```python
from build123d import *


with BuildPart() as part:
    # Sketch 1 → Revolve 1 (revolve)
    with BuildSketch(Plane.XY, mode=Mode.PRIVATE) as revolve_1_sk:
        with BuildLine():
            Line((18.75, 20), (18.75, 24))
            ThreePointArc((18.75, 24), (18.457106781, 24.707106781), (17.75, 25))
            Line((17.75, 25), (-16, 25))
            ThreePointArc((-16, 25), (-16.258819045, 24.965925826), (-16.5, 24.866025404))
            Line((-16.5, 24.866025404), (-18.25, 23.855662433))
            ThreePointArc((-18.25, 23.855662433), (-18.616025404, 23.489637029), (-18.75, 22.989637029))
            Line((-18.75, 22.989637029), (-18.75, 19.1))
            ThreePointArc((-18.75, 19.1), (-18.457106781, 18.392893219), (-17.75, 18.1))
            Line((-17.75, 18.1), (-16, 18.1))
            Line((-16, 18.1), (-16, 20))
            Line((-16, 20), (18.75, 20))
        make_face()
    revolve(revolve_1_sk.sketch.rotate(Axis((-18.75, 0, 0), (1, 0, 0)), 90), axis=Axis((-18.75, 0, 0), (1, 0, 0)))


solid = part.part
```
Could you check a few things on this model? Use its own coordinates, in mm. A direction names the side the tool comes from. Give positions to 0.01 mm unless a question says otherwise; leave off trailing zeros. Write each loop counter-clockwise with the first axis right and the second up, starting at its lowest first coordinate (ties: lowest second). Pieces come first, ordered by that corner, then holes. Notation, with made-up numbers: (50, 44) -> (78, 44) arc R12 ccw to (78, 66) -> close; hole circle Ø1 at (52, 68.25). An arc over 180 degrees is marked (long way). Write each question's results on one line, items separated by ' | '.
1. I want a section at A-A, the plane z = 0. Write out the boundary of the cut face in (x, y), then the cut area to 3 significant figures.
Check sheet entries:
outline: (-18.75, -22.99) arc R1 ccw to (-18.25, -23.86) -> (-16.5, -24.87) arc R1 ccw to (-16, -25) -> (17.75, -25) arc R1 ccw to (18.75, -24) -> (18.75, -20) -> (-16, -20) -> (-16, -18.1) -> (-17.75, -18.1) arc R1 ccw to (-18.75, -19.1) -> close; (-18.75, 19.1) arc R1 ccw to (-17.75, 18.1) -> (-16, 18.1) -> (-16, 20) -> (18.75, 20) -> (18.75, 24) arc R1 ccw to (17.75, 25) -> (-16, 25) arc R1 ccw to (-16.5, 24.87) -> (-18.25, 23.86) arc R1 ccw to (-18.75, 22.99) -> close | area: 381 mm²
2. Will these pins go through, and if not, where does the flat tip stop? pin 1 Ø12 at (x, y) = (-5, 19) entering from +Z; pin 2 Ø8 at (x, y) = (14, -9) entering from +Z; pin 3 Ø6 at (x, z) = (-2, 2.5) entering from +Y.
Check sheet entries:
pin 1: stops at z = 21.35 | pin 2: stops at z = 24.49 | pin 3: stops at y = 25
3. I want a section at C-C, the plane x = 14. Write out the boundary of the cut face in (y, z), then the cut area to 3 significant figures.
Check sheet entries:
outline: circle Ø50 at (0, 0); hole circle Ø40 at (0, 0) | area: 707 mm²
4. I need wall thicknesses on L1, parallel to Y at x = -1, z = 0; L2, parallel to Z at x = 9, y = 0.5 (3 decimals); L3, parallel to Y at x = -11.5, z = 8.5. Which ranges of each line are inside material? Lowest first, please.
Check sheet entries:
L1: y = -25 to -20, 20 to 25 | L2: z = -24.995 to -19.994, 19.994 to 24.995 | L3: y = -23.51 to -18.1, 18.1 to 23.51
5. If we mould it in two halves opening along Z, with no side actions, what happens to faces 1 (the flat face through (-16, 18, 5)), 2 (the flat face through (18.75, -20, 5)), 3 (the cylindrical face through (0.639, -7.509, 23.846))? For each: released by +Z, released by -Z, zero draft, split by the parting line, or undercut.
Check sheet entries:
face 1: undercut | face 2: zero draft | face 3: split by the parting line
6. On a 3-axis mill with a long thin cutter (end or side, diameter ignored), from which of +Z, -Z, +X, -X, +Y, -Y can I reach the whole of each face in a straight line? I mean faces 4 (the flat face through (-18.75, -19, -5)), 5 (the cylindrical face through (1.62, -0.88, -19.98)). Say none if no direction works.
Check sheet entries:
face 4: +Z, -Z, -X, +Y, -Y | face 5: +X
